Can you work these out from the model? Positions are in its coordinate system, mm. Face numbers are marked on the shaded views. A direction names the side the tool comes from. Coordinates: 2 decimals unless noted, no trailing zeros. Order: outer loops, then holes, each group sorted by start corner. A loop starts at its lowest first (then second) coordinate and runs counter-clockwise, first axis right, second up. Notation, with made-up numbers: (80, -18) -> (134, -18) arc R25 cw to (134, -1) -> close; hole circle Ø5 at (44, 2.25). An arc over 180 degrees is marked (long way). Return JSON: item names as keys, results as strings. Group by question number.
1) If we section it at B-B, the plane y = 0: Please give me the cut outline in (x, z).
2) Thinking about a two-plate mould opening in X: for the marked faces 4, 5 and 6, which applies, +X half, -X half, draft (parallel to the pull), parting line (faces both ways), or undercut?
3) If we section it at C-C, the plane x = 0: State how many separate pieces and enclosed holes the cut face has, then the cut area to 3 significant figures.
4) If we section it at D-D, the plane y = -28: Please give me the cut outline in (x, z), then the cut area to 3 significant figures.
5) If I drill on probe 1 along Y at (x, z) = (-15, 4.1); probe 2 along Y at (x, z) = (0, 4.4); probe 3 along X at (y, z) = (-18, 5.5), over which ranges is the centre line in solid material (lowest first)? Write a range as from..to.
6) For the marked faces 1, 2 and 3, which set-ups out of +Z, -Z, +X, -X, +Y, -Y let a thin tool reach every point of the face, with its end or its side?
7) For pin 1 (4 mm diameter, centred on x = -21.92, y = 0, fed in from +Z); pin 2 (2.5 mm diameter, centred on x = 11, y = -8.5, fed in from -Z), each with a flat end and sliding along its axis, tell me the tip position at first contact or that it passes through.
8) If we section it at A-A, the plane x = 22: Please give me the cut outline in (y, z), then the cut area to 3 significant figures.
from build123d import *

# Parameters (mm, degrees)
SKETCH_W        = 59.5
SKETCH_H        = 66
PAD_DEPTH       = 12
SKETCH001_R     = 3.3
POCKET_DEPTH    = 6
SKETCH002_R     = 3.3
SKETCH002_R_2   = 1.6
POCKET001_DEPTH = 6.001
SKETCH003_R     = 4
POCKET002_DEPTH = 59.501
SKETCH004_R     = 3.3
POCKET003_DEPTH = 5.5
POCKET004_DEPTH = 5.5
SKETCH006_R     = 11.5
POCKET005_DEPTH = 12.001
SKETCH007_W     = 9
SKETCH007_H     = 4
POCKET006_DEPTH = 26
FILLET_R        = 4
FILLET001_R     = 4
FILLET002_R     = 1
FILLET003_R     = 1


with BuildPart() as part:
    # Sketch → Pad (new body)
    with BuildSketch(Plane.XY):
        with Locations((-2.25, 0)):
            Rectangle(SKETCH_W, SKETCH_H)
    extrude(amount=PAD_DEPTH)

    # Sketch001 (on Face6 of Pad) → Pocket (cut)
    with BuildSketch(Plane.XY.offset(12)):
        with Locations((0, 21.92031)):
            Circle(SKETCH001_R)
        with Locations((-21.92031, 0)):
            Circle(SKETCH001_R)
        with Locations((21.92031, 0)):
            Circle(SKETCH001_R)
        with Locations((0, -21.92031)):
            Circle(SKETCH001_R)
        Polygon((-9.630642, 18.1), (-15, 21.2), (-20.369358, 18.1), (-20.369358, 11.9), (-15, 8.8), (-9.630642, 11.9), align=None)
        Polygon((20.369358, 18.1), (15, 21.2), (9.630642, 18.1), (9.630642, 11.9), (15, 8.8), (20.369358, 11.9), align=None)
        Polygon((-20.369358, -18.1), (-15, -21.2), (-9.630642, -18.1), (-9.630642, -11.9), (-15, -8.8), (-20.369358, -11.9), align=None)
        Polygon((20.369358, -11.9), (15, -8.8), (9.630642, -11.9), (9.630642, -18.1), (15, -21.2), (20.369358, -18.1), align=None)
    extrude(amount=-POCKET_DEPTH, mode=Mode.SUBTRACT)

    # Sketch002 (on Face41 of Pocket) → Pocket001 (cut, through all)
    with BuildSketch(Plane.XY.offset(6)):
        with Locations((-15, 15)):
            Circle(SKETCH002_R)
        with Locations((0, 21.92031)):
            Circle(SKETCH002_R_2)
        with Locations((15, 15)):
            Circle(SKETCH002_R)
        with Locations((-15, -15)):
            Circle(SKETCH002_R)
        with Locations((15, -15)):
            Circle(SKETCH002_R)
        with Locations((0, -21.92031)):
            Circle(SKETCH002_R_2)
        with Locations((21.92031, 0)):
            Circle(SKETCH002_R_2)
        with Locations((-21.92031, 0)):
            Circle(SKETCH002_R_2)
    extrude(amount=-POCKET001_DEPTH, mode=Mode.SUBTRACT)

    # Sketch003 (on Face3 of Pocket001) → Pocket002 (cut, through all)
    with BuildSketch(Plane.YZ.offset(27.5)):
        with Locations((-28, 0)):
            Circle(SKETCH003_R)
        with Locations((28, 0)):
            Circle(SKETCH003_R)
    extrude(amount=-POCKET002_DEPTH, mode=Mode.SUBTRACT)

    # Sketch004 (on Face2 of Pocket002) → Pocket003 (cut)
    with BuildSketch(Plane(origin=(-32, 0, 0), x_dir=(0, -1, 0), z_dir=(-1, 0, 0))):
        with Locations((-15, 0)):
            Circle(SKETCH004_R)
        with Locations((15, 0)):
            Circle(SKETCH004_R)
    extrude(amount=-POCKET003_DEPTH, mode=Mode.SUBTRACT)

    # Sketch005 (on Face42 of Pocket003) → Pocket004 (cut)
    with BuildSketch(Plane(origin=(-26.5, 0, 0), x_dir=(0, -1, 0), z_dir=(-1, 0, 0))):
        Polygon((-9.630642, 3.1), (-15, 6.2), (-20.369358, 3.1), (-20.369358, -3.1), (-15, -6.2), (-9.630642, -3.1), align=None)
        Polygon((9.630642, -3.1), (15, -6.2), (20.369358, -3.1), (20.369358, 3.1), (15, 6.2), (9.630642, 3.1), align=None)
    extrude(amount=-POCKET004_DEPTH, mode=Mode.SUBTRACT)

    # Sketch006 (on Face5 of Pocket004) → Pocket005 (cut, through all)
    with BuildSketch(Plane.XY.offset(12)):
        Circle(SKETCH006_R)
    extrude(amount=-POCKET005_DEPTH, mode=Mode.SUBTRACT)

    # Sketch007 (on Face3 of Pocket005) → Pocket006 (cut)
    with BuildSketch(Plane.YZ.offset(27.5)):
        with Locations((-7, 2)):
            Rectangle(SKETCH007_W, SKETCH007_H)
        with Locations((7, 2)):
            Rectangle(SKETCH007_W, SKETCH007_H)
    extrude(amount=-POCKET006_DEPTH, mode=Mode.SUBTRACT)

    # Fillet
    fillet_edges = [part.edges().sort_by_distance(p)[0] for p in [
        (-2.25, -33, 12),
    ]]
    fillet(fillet_edges, radius=FILLET_R)

    # Fillet001
    fillet001_edges = [part.edges().sort_by_distance(p)[0] for p in [
        (-2.25, 33, 12),
    ]]
    fillet(fillet001_edges, radius=FILLET001_R)

    # Fillet002
    fillet002_edges = [part.edges().sort_by_distance(p)[0] for p in [
        (-32, 0, 12),
    ]]
    fillet(fillet002_edges, radius=FILLET002_R)

    # Fillet003
    fillet003_edges = [part.edges().sort_by_distance(p)[0] for p in [
        (27.5, 0, 12),
    ]]
    fillet(fillet003_edges, radius=FILLET003_R)


solid = part.part
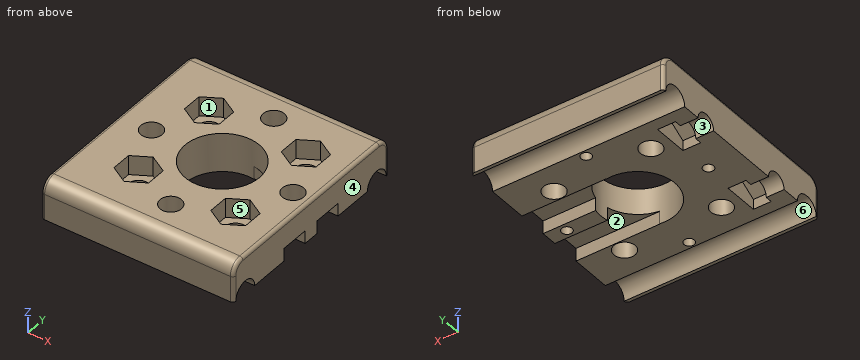
Result sheet:
{
 "1": {"outline": "(-32, 0) -> (-23.52, 0) -> (-23.52, 6) -> (-25.22, 6) -> (-25.22, 12) -> (-31, 12) arc R1 ccw to (-32, 11) -> close; (-20.32, 0) -> (-11.5, 0) -> (-11.5, 12) -> (-18.62, 12) -> (-18.62, 6) -> (-20.32, 6) -> close; (11.5, 0) -> (20.32, 0) -> (20.32, 6) -> (18.62, 6) -> (18.62, 12) -> (11.5, 12) -> close; (23.52, 0) -> (27.5, 0) -> (27.5, 11) arc R1 ccw to (26.5, 12) -> (25.22, 12) -> (25.22, 6) -> (23.52, 6) -> close"},
 "2": {"face 4": "+X half", "face 5": "undercut", "face 6": "draft"},
 "3": {"separate pieces": "4", "enclosed holes": "0", "area": "341 mm2"},
 "4": {"outline": "(-32, 4) -> (27.5, 4) -> (27.5, 11) arc R1 ccw to (26.5, 12) -> (-31, 12) arc R1 ccw to (-32, 11) -> close", "area": "476 mm2"},
 "5": {"probe 1": "y = -33..-18.3, -11.7..11.7, 18.3..33", "probe 2": "y = -33..-23.52, -20.32..-11.5, 11.5..20.32, 23.52..33", "probe 3": "x = -32..-16.37, -13.63..13.63, 16.37..27.5"},
 "6": {"face 1": "+Z", "face 2": "-Z, +X", "face 3": "-Z, -X"},
 "7": {"pin 1": "stops at z = 6", "pin 2": "stops at z = 4"},
 "8": {"outline": "(-33, 0) -> (-32, 0) arc R4 cw to (-24, 0) -> (-11.5, 0) -> (-11.5, 4) -> (-2.5, 4) -> (-2.5, 0) -> (-1.6, 0) -> (-1.6, 6) -> (-3.3, 6) -> (-3.3, 12) -> (-29, 12) arc R4 ccw to (-33, 8) -> close; (1.6, 0) -> (2.5, 0) -> (2.5, 4) -> (11.5, 4) -> (11.5, 0) -> (24, 0) arc R4 cw to (32, 0) -> (33, 0) -> (33, 8) arc R4 ccw to (29, 12) -> (3.3, 12) -> (3.3, 6) -> (1.6, 6) -> close", "area": "604 mm2"}
}
